from build123d import *

# Parameters (mm, degrees)
F0_W     = 1739.9
F0_H     = 19.05
F1_DEPTH = 431.8
F2_R     = 3.175
F3_DEPTH = 9.525
F4_W     = 9.525
F4_H     = 76.2
F4_W_2   = 234.95
F4_H_2   = 234.95
F5_DEPTH = 3.175


with BuildPart() as f1:
    # F0 (on Front) → F1 (new body)
    with BuildSketch(Plane.XZ):
        with Locations((869.95, 9.525)):
            Rectangle(F0_W, F0_H)
    extrude(amount=-F1_DEPTH)

    # F2 (on face) → F3 (cut)
    with BuildSketch(Plane(origin=(0, 0, 0), x_dir=(1, 0, 0), z_dir=(0, 0, -1))):
        with Locations((1730.375, -381)):
            Circle(F2_R)
        with Locations((1730.375, -215.9)):
            Circle(F2_R)
        with Locations((1730.375, -50.8)):
            Circle(F2_R)
        with Locations((9.525, -381)):
            Circle(F2_R)
        with Locations((9.525, -215.9)):
            Circle(F2_R)
        with Locations((9.525, -50.8)):
            Circle(F2_R)
        with Locations((1384.3, -50.8)):
            Circle(F2_R)
        with Locations((1384.3, -279.4)):
            Circle(F2_R)
        with Locations((698.5, -50.8)):
            Circle(F2_R)
        with Locations((355.6, -279.4)):
            Circle(F2_R)
        with Locations((698.5, -279.4)):
            Circle(F2_R)
        with Locations((1041.4, -50.8)):
            Circle(F2_R)
        with Locations((1041.4, -279.4)):
            Circle(F2_R)
        with Locations((355.6, -50.8)):
            Circle(F2_R)
    extrude(amount=-F3_DEPTH, mode=Mode.SUBTRACT)

    # F4 (on face) → F5 (cut)
    with BuildSketch(Plane(origin=(0, 0, 0), x_dir=(1, 0, 0), z_dir=(0, 0, -1))):
        with Locations((1677.9875, -330.2)):
            Rectangle(F4_W, F4_H)
        Polygon((1673.225, -292.1), (1682.75, -292.1), (1682.75, -38.1), (1428.75, -38.1), (1428.75, -292.1), align=None)
        with Locations((1555.75, -165.1)):
            Rectangle(F4_W_2, F4_H_2, mode=Mode.SUBTRACT)
        with Locations((1335.0875, -330.2)):
            Rectangle(F4_W, F4_H)
        Polygon((1330.325, -292.1), (1339.85, -292.1), (1339.85, -38.1), (1085.85, -38.1), (1085.85, -292.1), align=None)
        with Locations((1212.85, -165.1)):
            Rectangle(F4_W_2, F4_H_2, mode=Mode.SUBTRACT)
        with Locations((992.1875, -330.2)):
            Rectangle(F4_W, F4_H)
        Polygon((987.425, -292.1), (996.95, -292.1), (996.95, -38.1), (742.95, -38.1), (742.95, -292.1), align=None)
        with Locations((869.95, -165.1)):
            Rectangle(F4_W_2, F4_H_2, mode=Mode.SUBTRACT)
        with Locations((649.2875, -330.2)):
            Rectangle(F4_W, F4_H)
        Polygon((644.525, -292.1), (654.05, -292.1), (654.05, -38.1), (400.05, -38.1), (400.05, -292.1), align=None)
        with Locations((527.05, -165.1)):
            Rectangle(F4_W_2, F4_H_2, mode=Mode.SUBTRACT)
        with Locations((306.3875, -330.2)):
            Rectangle(F4_W, F4_H)
        Polygon((301.625, -292.1), (311.15, -292.1), (311.15, -38.1), (57.15, -38.1), (57.15, -292.1), align=None)
        with Locations((184.15, -165.1)):
            Rectangle(F4_W_2, F4_H_2, mode=Mode.SUBTRACT)
    extrude(amount=-F5_DEPTH, mode=Mode.SUBTRACT)


solid = f1.part
Could you check a few things on this model? Use its own coordinates, in mm. Round coordinates to 2 decimals unless told otherwise and drop trailing zeros. Put each result on its own line as item: value. Start each with the question number.
(1) I need wall thicknesses on probe 1 along X at (y, z) = (215.9, 7); probe 2 along Y at (x, z) = (355.6, 6.5) (3 decimals); probe 3 along Z at (x, y) = (303.5, 67.5) (3 decimals). Which ranges of each line are inside material? Lowest first, please.
(2) Thinking about a two-plate mould opening in X: for faces 1 (the flat face through (536, 288, 3.175)), 2 (the flat face through (193, 288, 3.175)), 3 (the flat face through (183, 163, 0)), which applies, released by +X, released by -X, zero draft, split by the parting line, or undercut?
(3) Will this pin go through, and if not, where does the flat tip stop? pin 1 (5.5 mm diameter, centred on x = 1384.3, y = 50.8, fed in from -Z) (3 decimals).
Here are the results:
1. probe 1: x = 0 to 6.35, 12.7 to 1727.2, 1733.55 to 1739.9
1. probe 2: y = 0 to 47.625, 53.975 to 276.225, 282.575 to 431.8
1. probe 3: z = 3.175 to 19.05
2. face 1: undercut
2. face 2: undercut
2. face 3: zero draft
3. pin 1: stops at z = 9.525
